The figure shows three views and two pictorial views of one solid part (mm, origin at its lowest corner). Answer the questions. Coordinates: 2 decimals unless noted, no trailing zeros. Loops run counter-clockwise (first coordinate to the right, second up) from the corner with the lowest first, then second, coordinate; pieces in that order, holes last. Notation, with made-up numbers: (-21, 87) -> (-15, 87) arc R20 cw to (-15, 105) -> close; hole circle Ø10 at (4, -5.5). An arc over 180 degrees is marked (long way). Answer in a Markdown table with one row per item.
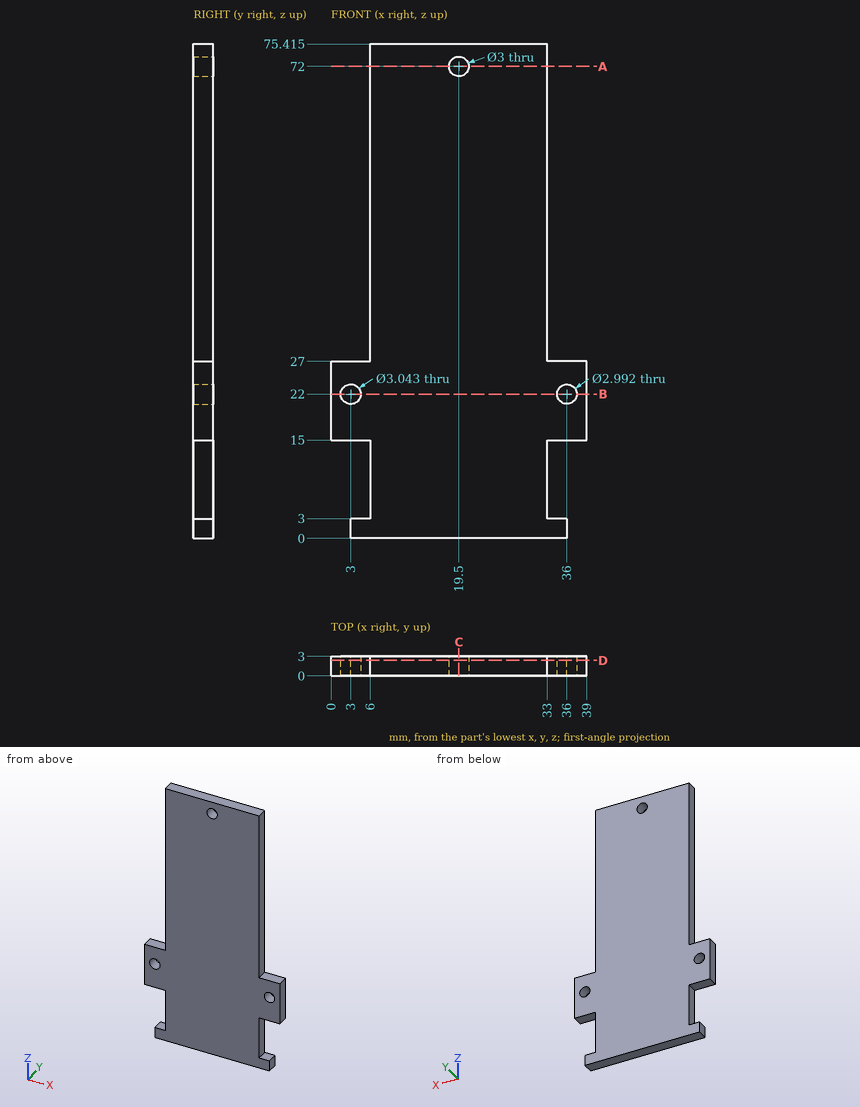
Item 1: Flat-ended cylindrical pins translate along their axes: pin 1 Ø0.9 at (y, z) = (1.5, 8) entering from +X; pin 2 Ø3.5 at (x, z) = (19.5, 72) entering from +Y. Find the tip coordinate at first contact, or state that the pin passes through.
Findings below:
| item | result |
|---|---|
| pin 1 | stops at x = 33 |
| pin 2 | stops at y = 3 |
Item 2: A cutting plane is placed at B-B, the plane z = 22. Determine the outline of the cut face in (x, y).
Findings below:
| item | result |
|---|---|
| outline | (0, 0) -> (1.48, 0) -> (1.48, 3) -> (0, 3) -> close; (4.52, 0) -> (34.5, 0) -> (34.5, 3) -> (4.52, 3) -> close; (37.5, 0) -> (39, 0) -> (39, 3) -> (37.5, 3) -> close |
Item 3: A cutting plane is placed at A-A, the plane z = 72. Determine the outline of the cut face in (x, y).
Findings below:
| item | result |
|---|---|
| outline | (6, 0) -> (18, 0) -> (18, 3) -> (6, 3) -> close; (21, 0) -> (33, 0) -> (33, 3) -> (21, 3) -> close |
Item 4: Find the intervals of material crossed by probe 1 along X at (y, z) = (1.95, 22); probe 2 along Z at (x, y) = (33.5, 2.3); probe 3 along X at (y, z) = (2.15, 64.5), in increasing order.
Findings below:
| item | result |
|---|---|
| probe 1 | x = 0 to 1.48, 4.52 to 34.5, 37.5 to 39 |
| probe 2 | z = 0 to 3, 15 to 27 |
| probe 3 | x = 6 to 33 |
Item 5: A cutting plane is placed at D-D, the plane y = 2.4. Determine the outline of the cut face in (x, z) (1 decimal).
Findings below:
| item | result |
|---|---|
| outline | (0, 15) -> (6, 15) -> (6, 3) -> (3, 3) -> (3, 0) -> (36, 0) -> (36, 3) -> (33, 3) -> (33, 15) -> (39, 15) -> (39, 27) -> (33, 27) -> (33, 75.4) -> (6, 75.4) -> (6, 27) -> (0, 27) -> close; hole circle Ø3 at (3, 22); hole circle Ø3 at (19.5, 72); hole circle Ø3 at (36, 22) |
Item 6: A cutting plane is placed at C-C, the plane x = 19.5. Determine the outline of the cut face in (y, z) (1 decimal), plus the area to 3 significant figures.
Findings below:
| item | result |
|---|---|
| outline | (0, 0) -> (3, 0) -> (3, 70.5) -> (0, 70.5) -> close; (0, 73.5) -> (3, 73.5) -> (3, 75.4) -> (0, 75.4) -> close |
| area | 217 mm2 |
